Check sheet for the modelled part. Datum: model origin and axes. Units: mm. Face numbers are marked on the shaded views. A direction names the side the tool comes from. Coordinates: 2 decimals unless noted, no trailing zeros. Loops run counter-clockwise (first coordinate to the right, second up) from the corner with the lowest first, then second, coordinate; pieces in that order, holes last. Notation, with made-up numbers: (35.25, 42) - (44.25, 42) arc R12 ccw to (44.25, 62) - close; hole circle Ø7 at (50, 70). An arc over 180 degrees is marked (long way). Write each question's results on one line, items separated by ' | '. Start each with the question number.
1. Cross-section at B-B (x = 5.25). Record the cut outline in (y, z).
2. Draft check along X on the marked faces 4, 5, 6 and 7. Enter one of: released by +X, released by -X, zero draft, split by the parting line, or undercut.
3. Thickness scan on line 1 (Y direction, x = 5.5, z = 1.65); line 2 (Y direction, x = 7, z = 2.7); line 3 (X direction, y = 7.5, z = 1.7). Record the ranges inside material, lowest first. Write a range as [from, to].
4. Cross-section at A-A (z = 1.05). Record the cut outline in (x, y) (1 decimal).
5. Cross-section at C-C (y = 9.5). Record the cut outline in (x, z).
6. Tool access check on the marked faces 1, 2 and 3. Record the directions out of +Z, -Z, +X, -X, +Y, -Y that give a thin tool (end or side, any length) a straight path to the whole face; none if there is none.
7. Gauge pin test, flat end, axial feed: P1, Ø1.1, axis at y = 7, z = 1, coming from the -X side. Record the tip position at first contact, or that the pin passes through.
8. Cross-section at D-D (x = -8). Record the cut outline in (y, z), and give its area (3 significant figures).
Autodesk Inventor part; units mm, degrees
ref_plane "YZ Plane" through (0, 0, 0) normal (1, 0, 0) x (0, 1, 0)
ref_plane "XZ Plane" through (0, 0, 0) normal (0, 1, 0) x (-1, 0, 0)
ref_plane "XY Plane" through (0, 0, 0) normal (0, 0, 1) x (1, 0, 0)
sketch "Sketch1" plane through (0, 0, 0) normal (0, 0, 1) x (1, 0, 0)
  arc A0 (1.4995, 7.5) -> (-1.385, 6.9228) centre (-0.0005, 7.5) ccw
  arc A1 (-1.3846, -6.9231) -> (1.5, -7.5) centre (0, -7.5) ccw
  arc A2 (-10.3524, -1.1528) -> (-10.356, 1.1198) centre (-12, -0.0191) ccw
  arc A3 (10.1341, 4.2778) -> (-10.6479, 2.7607) centre (0, 0) ccw
  arc A4 (-10.6391, -2.7946) -> (10.1341, -4.2778) centre (0, 0) ccw
  arc A5 (-10.6479, 2.7607) -> (-10.356, 1.1198) centre (-8.7119, 2.2588) ccw
  arc A6 (-10.3524, -1.1528) -> (-10.6391, -2.7946) centre (-8.7047, -2.2865) ccw
  line L0 (-1, -5) -> (-1, 4.9988)
  arc A7 (-1, 4.9988) -> (-1.385, 6.9228) centre (-6, 4.9988) ccw
  arc A8 (-1.3846, -6.9231) -> (-1, -5) centre (-6, -5) ccw
  line L1 (1.4995, 7.5) -> (1.4995, 6.5)
  line L2 (1.4995, -6.5) -> (1.4995, -7.5382)
  line L3 (6.4995, -1.5) -> (8.2916, -1.5)
  line L4 (6.4995, 1.5) -> (8.2916, 1.5)
  arc A9 (6.4995, -1.5) -> (1.4995, -6.5) centre (6.4995, -6.5) ccw
  arc A10 (1.4995, 6.5) -> (6.4995, 1.5) centre (6.4995, 6.5) ccw
  arc A11 (10.1341, -4.2778) -> (8.2916, -1.5) centre (8.2916, -3.5) ccw
  arc A12 (8.2916, 1.5) -> (10.1341, 4.2778) centre (8.2916, 3.5) ccw
  point P0 (10.8972, -1.5)
  point P1 (10.8972, 1.5)
  point P2 (1.4995, 1.5)
  point P3 (1.4995, -1.5)
  point P4 (-1, -6.382)
  point P5 (-1, 6.3815)
  dimension "d5" = 3
  dimension "d6" = 3
  dimension "d7" = 15
  dimension "d18" = 7.5
  dimension "d20" = 4
  dimension "d21" = 12
  dimension "d22" = 2
  dimension "d26" = 5
  dimension "d27" = 5
  dimension "d28" = 2
extrude "Extrusion2" add sketch "Sketch1" along normal blind 3
properties part number "Middle Endcap080813" material "Polycarbonate, Clear"
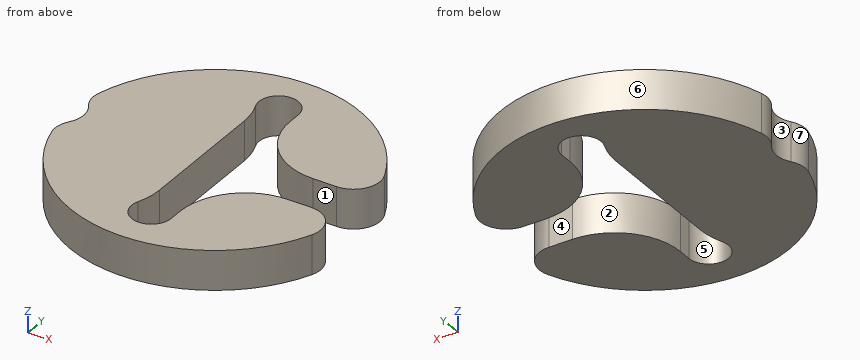
Established:
1) outline: (-9.67, 0) - (-1.66, 0) - (-1.66, 3) - (-9.67, 3) - close; (1.66, 0) - (9.67, 0) - (9.67, 3) - (1.66, 3) - close
2) face 4: zero draft | face 5: undercut | face 6: split by the parting line | face 7: released by -X
3) line 1: [-9.53, -1.6], [1.6, 9.53] | line 2: [-8.49, -1.5], [1.5, 8.49] | line 3: [-8.05, -1.5], [1.5, 8.05]
4) outline: (-10.6, -2.8) arc R11 ccw to (10.1, -4.3) arc R2 ccw to (8.3, -1.5) - (6.5, -1.5) arc R5 ccw to (1.5, -6.5) - (1.5, -7.5) arc R1.5 cw (long way) to (-1.4, -6.9) arc R5 ccw to (-1, -5) - (-1, 5) arc R5 ccw to (-1.4, 6.9) arc R1.5 cw (long way) to (1.5, 7.5) - (1.5, 6.5) arc R5 ccw to (6.5, 1.5) - (8.3, 1.5) arc R2 ccw to (10.1, 4.3) arc R11 ccw to (-10.6, 2.8) arc R2 ccw to (-10.4, 1.1) arc R2 cw to (-10.4, -1.2) arc R2 ccw to start
5) outline: (-5.55, 0) - (5.55, 0) - (5.55, 3) - (-5.55, 3) - close
6) face 1: +Z, -Z, +X | face 2: +Z, -Z | face 3: +Z, -Z, -X
7) P1: x = -8.91
8) outline: (-7.55, 0) - (7.55, 0) - (7.55, 3) - (-7.55, 3) - close | area: 45.3 mm^2
